Here's how the part is built. I have some questions about the finished solid (model axes, mm). Coordinates: 2 decimals unless noted, no trailing zeros. Loops run counter-clockwise (first coordinate to the right, second up) from the corner with the lowest first, then second, coordinate; pieces in that order, holes last.
from build123d import *

# Parameters (mm, degrees)
SKETCH_R             = 17.86
PAD_DEPTH            = 1.6
SKETCH001_R          = 4.765
PAD001_DEPTH         = 7.96
SKETCH002_R          = 2.15
POCKET_DEPTH         = 9.561
SKETCH003_R          = 1.6
POCKET001_DEPTH      = 5
POCKET001_DEPTH_BACK = -5
SKETCH004_R          = 2.15
POCKET002_DEPTH      = 112.385713
POLARPATTERN_COUNT   = 8


with BuildPart() as part:
    # Sketch → Pad (new body)
    with BuildSketch(Plane.XY):
        Circle(SKETCH_R)
    extrude(amount=PAD_DEPTH)

    # Sketch001 (on Face3 of Pad) → Pad001 (join)
    with BuildSketch(Plane.XY.offset(1.6)):
        Circle(SKETCH001_R)
    extrude(amount=PAD001_DEPTH)

    # Sketch002 (on Face5 of Pad001) → Pocket (cut, through all)
    with BuildSketch(Plane.XY.offset(9.56)):
        Circle(SKETCH002_R)
    extrude(amount=-POCKET_DEPTH, mode=Mode.SUBTRACT)

    # Sketch003 (on DatumPlane) → Pocket001 (cut, two sides)
    with BuildSketch(Plane(origin=(0, 0, 0), x_dir=(0.92388, 0.382683, 0), z_dir=(0.382683, -0.92388, 0))) as pocket001_sk:
        with Locations((0, 5.57)):
            Circle(SKETCH003_R)
    extrude(amount=-POCKET001_DEPTH, mode=Mode.SUBTRACT)
    extrude(pocket001_sk.sketch, amount=-POCKET001_DEPTH_BACK, mode=Mode.SUBTRACT)

    # Sketch004 → Pocket002 (cut, through all)
    with BuildSketch(Plane.XY):
        with Locations((0, 12.7)):
            Circle(SKETCH004_R)
    pocket002 = extrude(amount=POCKET002_DEPTH, mode=Mode.SUBTRACT)

    # PolarPattern: Pocket002 ×8 about axis
    polarpattern_axis = Axis((0, 0, 0), (0, 0, 1))
    for i in range(1, POLARPATTERN_COUNT):
        add(pocket002.rotate(polarpattern_axis, i * 360 / POLARPATTERN_COUNT), mode=Mode.SUBTRACT)


solid = part.part
Q1. Suppose I cut it at D-D on y = 10. Write out the boundary of the cut face in (x, z), and give its area (3 significant figures).
Q2. Suppose I cut it at B-B on x = -14. Write out the boundary of the cut face in (y, z).
Q3. Suppose I cut it at C-C on z = 6.75. Write out the boundary of the cut face in (x, y) (3 decimals).
Q4. Suppose I cut it at A-A on y = 0. Write out the boundary of the cut face in (x, z) (3 decimals), and give its area (3 significant figures).
Q5. Will these pins go through, and if not, where does the flat tip stop? P1, Ø5.5, axis at x = -8.98, y = -8.98, coming from the +Z side; P2, Ø2, axis at x = 2.5, z = 2.5, coming from the -Y side.
Q6. Please list where these lines run through material, in increasing order: probe 1 along Y at (x, z) = (0, 0.95); probe 2 along Y at (x, z) = (12.7, 1.15); probe 3 along Z at (x, y) = (-6, 4.5).
Q7. We'd pull the mould along X, two halves only. Please class faces 1 (the cylindrical face through (-4.76, 0.21, 5.52)), 2 (the cylindrical face through (9.26, -6.85, 0.79)), 3 (the flat face through (4, -4, 1.6)): pulls with the +X half, pulls with the -X half, needs draft (parallel to the pull), parting line crosses it, or undercut.
Check values:
1. outline: (-14.8, 0) - (-10.87, 0) - (-10.87, 1.6) - (-14.8, 1.6) - close; (-7.09, 0) - (7.09, 0) - (7.09, 1.6) - (-7.09, 1.6) - close; (10.87, 0) - (14.8, 0) - (14.8, 1.6) - (10.87, 1.6) - close
1. area: 35.2 mm2
2. outline: (-11.09, 0) - (-1.71, 0) - (-1.71, 1.6) - (-11.09, 1.6) - close; (1.71, 0) - (11.09, 0) - (11.09, 1.6) - (1.71, 1.6) - close
3. outline: (-2.774, 3.874) arc R4.765 ccw to (0.778, -4.701) - (-0.287, -2.131) arc R2.15 cw to (-1.71, 1.304) - close; (-0.778, 4.701) - (0.287, 2.131) arc R2.15 cw to (1.71, -1.304) - (2.774, -3.874) arc R4.765 ccw to start
4. outline: (-17.86, 0) - (-14.85, 0) - (-14.85, 1.6) - (-17.86, 1.6) - close; (-10.55, 0) - (-2.15, 0) - (-2.15, 9.56) - (-4.765, 9.56) - (-4.765, 1.6) - (-10.55, 1.6) - close; (2.15, 0) - (10.55, 0) - (10.55, 1.6) - (4.765, 1.6) - (4.765, 9.56) - (2.15, 9.56) - close; (14.85, 0) - (17.86, 0) - (17.86, 1.6) - (14.85, 1.6) - close
4. area: 78.1 mm2
5. P1: stops at z = 1.6
5. P2: stops at y = -17.74
6. probe 1: y = -17.86 to -14.85, -10.55 to -2.15, 2.15 to 10.55, 14.85 to 17.86
6. probe 2: y = -12.56 to -2.15, 2.15 to 12.56
6. probe 3: z = 0 to 1.6
7. face 1: parting line crosses it
7. face 2: undercut
7. face 3: needs draft
